Could you check a few things on this model? Use its own coordinates, in mm. A direction names the side the tool comes from. Coordinates: 2 decimals unless noted, no trailing zeros. Loops run counter-clockwise (first coordinate to the right, second up) from the corner with the lowest first, then second, coordinate; pieces in that order, holes last. Notation, with made-up numbers: (46, 39.25) - (82, 39.25) arc R14 cw to (82, 43.25) - close; hole circle Ø4 at (-29, 86.5). An arc over 180 degrees is marked (long way). Use CSV: the item, a comma, the result in double quotes.
from build123d import *

# Parameters (mm, degrees)
SKETCH3_W           = 508
SKETCH3_H           = 111.76
BOSS_EXTRUDE1_DEPTH = 63.5
CUT_EXTRUDE1_START  = 6.35
SKETCH2_W           = 102.108
SKETCH2_H           = 102.108
CUT_EXTRUDE1_DEPTH  = 111.76
SKETCH4_R           = 50.8
CUT_EXTRUDE2_DEPTH  = 156.718
SKETCH5_R           = 43.18
CUT_EXTRUDE3_DEPTH  = 355.6
SKETCH6_W           = 266.7
SKETCH6_H           = 101.6
CUT_EXTRUDE4_DEPTH  = 50.8
SKETCH8_OUTSIDE_W   = 614.802
SKETCH8_OUTSIDE_H   = 218.562
CUT_EXTRUDE5_DEPTH  = 174.244
SKETCH9_W           = 25.4
SKETCH9_H           = 60.96
BOSS_EXTRUDE2_DEPTH = 10.16
SKETCH10_R          = 3.5
CUT_EXTRUDE6_DEPTH  = 93.98
SKETCH10_3_R        = 5.5
CUT_EXTRUDE7_DEPTH  = 45.72
SKETCH12_R          = 3.5
CUT_EXTRUDE8_DEPTH  = 93.98
SKETCH12_3_R        = 5.5
CUT_EXTRUDE9_DEPTH  = 7.5


with BuildPart() as part:
    # Sketch3 → Boss-Extrude1 (new body)
    with BuildSketch(Plane(origin=(0, 0, 0), x_dir=(1, 0, 0), z_dir=(0, 1, 0))):
        with Locations((203.2, 36.195)):
            Rectangle(SKETCH3_W, SKETCH3_H)
    extrude(amount=BOSS_EXTRUDE1_DEPTH)

    # Sketch2 → Cut-Extrude1 (cut)
    with BuildSketch(Plane(origin=(0, 0, 0), x_dir=(1, 0, 0), z_dir=(0, 1, 0)).offset(CUT_EXTRUDE1_START)):
        with Locations((400.05, 36.195)):
            Rectangle(SKETCH2_W, SKETCH2_H)
    extrude(amount=CUT_EXTRUDE1_DEPTH, mode=Mode.SUBTRACT)

    # Sketch4 → Cut-Extrude2 (cut)
    with BuildSketch(Plane.XY.offset(19.685)):
        with Locations((317.5, 63.5)):
            Circle(SKETCH4_R)
        Polygon((457.2, 12.7), (317.5, 12.7), (266.7, 63.5), (457.2, 63.5), align=None)
    extrude(amount=-CUT_EXTRUDE2_DEPTH, mode=Mode.SUBTRACT)

    # Sketch5 → Cut-Extrude3 (cut)
    with BuildSketch(Plane(origin=(0, 0, 0), x_dir=(0, 0, -1), z_dir=(1, 0, 0))):
        with Locations((36.195, 63.5)):
            Circle(SKETCH5_R)
    extrude(amount=CUT_EXTRUDE3_DEPTH, mode=Mode.SUBTRACT)

    # Sketch6 → Cut-Extrude4 (cut)
    with BuildSketch(Plane(origin=(0, 63.5, 0), x_dir=(1, 0, 0), z_dir=(0, 1, 0))):
        with Locations((87.63, 36.195)):
            Rectangle(SKETCH6_W, SKETCH6_H)
    extrude(amount=-CUT_EXTRUDE4_DEPTH, mode=Mode.SUBTRACT)

    # Sketch7 → Cut-Revolve1 (revolve, cut)
    with BuildSketch(Plane(origin=(0, 63.5, 0), x_dir=(1, 0, 0), z_dir=(0, 1, 0))):
        with BuildLine():
            Line((233.68, -13.805), (237.541436971, -13.805))
            ThreePointArc((237.541436971, -13.805), (238.359341863, -10.401680901), (239.119500346, -6.985))
            Line((239.119500346, -6.985), (233.68, -6.985))
            Line((233.68, -6.985), (233.68, -13.805))
        make_face()
    revolve(axis=Axis((-45.72, 63.5, -36.195), (1, 0, 0)), mode=Mode.SUBTRACT)

    # Sketch8 outside → Cut-Extrude5 (cut)
    with BuildSketch(Plane.XZ):
        with Locations((203.2, -36.195)):
            Rectangle(SKETCH8_OUTSIDE_W, SKETCH8_OUTSIDE_H)
        Polygon((248.92, 19.685), (248.92, -5.715), (274.32, -5.715), (274.32, -66.675), (248.92, -66.675), (248.92, -92.075), (493.448726159, -149.556417416), (493.448726159, 67.99660497), align=None, mode=Mode.SUBTRACT)
    extrude(amount=-CUT_EXTRUDE5_DEPTH, mode=Mode.SUBTRACT)

    # Sketch9 → Boss-Extrude2 (add)
    with BuildSketch(Plane.XZ):
        with Locations((261.62, -36.195)):
            Rectangle(SKETCH9_W, SKETCH9_H)
    extrude(amount=-BOSS_EXTRUDE2_DEPTH)

    # Sketch10 → Cut-Extrude6 (cut)
    with BuildSketch(Plane.XZ):
        with Locations(Location((258.9149, -84.963, 0), (0, 0, 270))):
            Circle(SKETCH10_R)
        with Locations(Location((258.9149, 12.573, 0), (0, 0, 270))):
            Circle(SKETCH10_R)
    extrude(amount=-CUT_EXTRUDE6_DEPTH, mode=Mode.SUBTRACT)

    # Sketch10_3 → Cut-Extrude7 (cut)
    with BuildSketch(Plane.XZ):
        with Locations(Location((258.9149, 12.573, 0), (0, 0, 270))):
            Circle(SKETCH10_3_R)
        with Locations(Location((258.9149, -84.963, 0), (0, 0, 270))):
            Circle(SKETCH10_3_R)
    extrude(amount=-CUT_EXTRUDE7_DEPTH, mode=Mode.SUBTRACT)

    # Sketch12 → Cut-Extrude8 (cut)
    with BuildSketch(Plane.XZ):
        with Locations(Location((261.62, -36.195, 0), (0, 0, 270))):
            Circle(SKETCH12_R)
    extrude(amount=-CUT_EXTRUDE8_DEPTH, mode=Mode.SUBTRACT)

    # Sketch12_3 → Cut-Extrude9 (cut)
    with BuildSketch(Plane.XZ):
        with Locations(Location((261.62, -36.195, 0), (0, 0, 270))):
            Circle(SKETCH12_3_R)
    extrude(amount=-CUT_EXTRUDE9_DEPTH, mode=Mode.SUBTRACT)


solid = part.part
(1) Please list where these lines run through material, in increasing order: line 1 (X direction, y = 6.5, z = -1); line 2 (Y direction, x = 365.5, z = -47); line 3 (X direction, y = 41.5, z = 12.5).
Computed:
line 1,"x = 248.92 to 349, 451.1 to 457.2"
line 2,"y = 0 to 6.35"
line 3,"x = 248.92 to 253.42, 264.41 to 271.71"
(2) Will these pins go through, and if not, where does the flat tip stop? pin 1 (12 mm diameter, centred on x = 397.5, z = -45.5, fed in from -Y); pin 2 (12 mm diameter, centred on y = 26.5, z = -3, fed in from +X); pin 3 (12.5 mm diameter, centred on x = 268, z = -30, fed in from +Y); pin 4 (10 mm diameter, centred on y = 19, z = -54, fed in from -X).
Computed:
pin 1,"stops at y = 0"
pin 2,"stops at x = 290.45"
pin 3,"stops at y = 10.16"
pin 4,"stops at x = 274.32"
(3) Suppose I cut it at C-C (x = 416.5). Write out the boundary of the cut face in (y, z) (3 decimals), plus the area to 3 significant figures.
Computed:
outline,"(0, -92.075) - (12.7, -92.075) - (12.7, -87.249) - (6.35, -87.249) - (6.35, 14.859) - (12.7, 14.859) - (12.7, 19.685) - (0, 19.685) - close"
area,"771 mm²"
(4) Suppose I cut it at A-A (y = 50.5). Write out the boundary of the cut face in (x, z) (3 decimals).
Computed:
outline,"(248.92, -92.075) - (268.392, -92.075) - (268.392, -77.372) - (248.92, -77.372) - close; (248.92, 4.982) - (268.392, 4.982) - (268.392, 19.685) - (248.92, 19.685) - close; hole circle Ø7 at (258.915, -84.963); hole circle Ø7 at (258.915, 12.573)"
(5) Suppose I cut it at B-B (z = -37). Write out the boundary of the cut face in (x, y).
Computed:
outline,"(248.92, 0) - (256.18, 0) - (256.18, 7.5) - (258.21, 7.5) - (258.21, 10.16) - (248.92, 10.16) - close; (265.03, 7.5) - (267.06, 7.5) - (267.06, 0) - (457.2, 0) - (457.2, 12.7) - (451.1, 12.7) - (451.1, 6.35) - (349, 6.35) - (349, 12.7) - (317.5, 12.7) arc R50.8 cw to (290.73, 20.33) - (274.32, 20.33) - (274.32, 10.16) - (265.03, 10.16) - close"
(6) Suppose I cut it at D-D (y = 16.5). Write out the boundary of the cut face in (x, z) (3 decimals), plus the area to 3 significant figures.
Computed:
outline,"(248.92, -92.075) - (298.222, -92.075) - (298.222, 19.685) - (248.92, 19.685) - (248.92, -5.715) - (274.32, -5.715) - (274.32, -66.675) - (248.92, -66.675) - close; hole circle Ø11 at (258.915, -84.963); hole circle Ø11 at (258.915, 12.573)"
area,"3,770 mm²"
(7) Thinking about a two-plate mould opening in X: for faces 1 (the face through (399, 6.35, -37)), 2 (the face through (295.526, 17.698, -35.413)), 3 (the face through (255.7, 63.5, -87.2)), which applies, +X half, -X half, draft (parallel to the pull), parting line (faces both ways), or undercut?
Computed:
face 1,"undercut"
face 2,"+X half"
face 3,"draft"
(8) Which directions (+Z, -Z, +X, -X, +Y, -Y) give clear straight access to the entire face, cutting with the end or side of a thin tool? Please do faces 4 (the face through (258.273, 3.698, -31.83)), 5 (the face through (451.104, 9, -35)), 6 (the face through (322, 10, 19.685)), 7 (the face through (262, 21, -66.675)).
Computed:
face 4,"-Y"
face 5,"+Y"
face 6,"+Z, +X, -X, +Y, -Y"
face 7,"-X, +Y"
